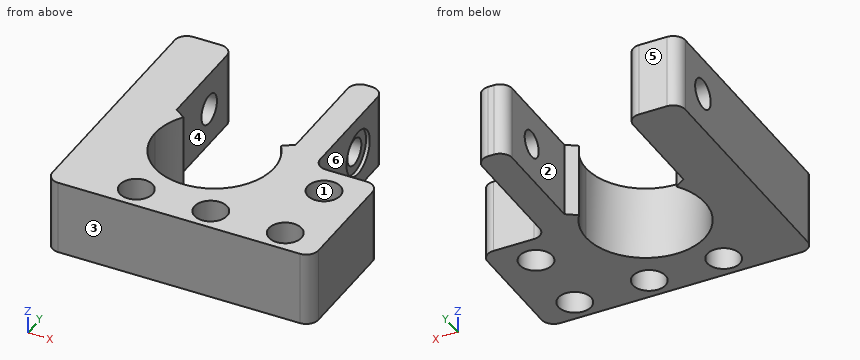
from build123d import *

# Parameters (mm, degrees)
CYLINDER011012_R               = 1.8
CYLINDER011012_DEPTH           = 20
CYLINDER011013_R               = 3
CYLINDER011013_DEPTH           = 20
CYLINDER011010_R               = 2.2
CYLINDER011010_DEPTH           = 100
ARRAY008_X_COUNT               = 3
ARRAY008_X_PITCH               = 10
ARRAY008_Y_COUNT               = 3
ARRAY008_Y_PITCH               = 10
CYLINDER011011_R               = 2
CYLINDER011011_DEPTH           = 20
CYLINDER011014_R               = 8
CYLINDER011014_DEPTH           = 10
CYLINDER011015_W               = 11
CYLINDER011015_H               = 10
CYLINDER011015_ANGLE           = 250
CYLINDER011015_PLACEMENT_ANGLE = 145
PAD_DEPTH                      = 10


with BuildPart() as bolt_hole001:
    # Cylinder011012 → Cylinder011012 (new body)
    with BuildSketch(Plane(origin=(-1, 14, 5), x_dir=(0, 0, -1), z_dir=(1, 0, 0))):
        Circle(CYLINDER011012_R)
    extrude(amount=CYLINDER011012_DEPTH)


with BuildPart() as bolt_head_hole:
    # Cylinder011013 → Cylinder011013 (new body)
    with BuildSketch(Plane(origin=(11.5, 14, 5), x_dir=(0, 0, -1), z_dir=(1, 0, 0))):
        Circle(CYLINDER011013_R)
    extrude(amount=CYLINDER011013_DEPTH)


with BuildPart() as general_insert_hole_array:
    # Cylinder011010 → Cylinder011010 (new body)
    with BuildSketch(Plane.XY):
        Circle(CYLINDER011010_R)
    extrude(amount=CYLINDER011010_DEPTH)

    # Array008 X: general insert hole array ×3


with BuildPart() as general_insert_hole_array_1:
    add(general_insert_hole_array.part)
    with Locations(*[(i * ARRAY008_X_PITCH, 0, 0) for i in range(1, ARRAY008_X_COUNT)]):
        add(general_insert_hole_array.part)

    # Array008 Y: general insert hole array ×3


with BuildPart() as general_insert_hole_array_2:
    add(general_insert_hole_array_1.part)
    with Locations(*[(0, i * ARRAY008_Y_PITCH, 0) for i in range(1, ARRAY008_Y_COUNT)]):
        add(general_insert_hole_array_1.part)


with BuildPart() as general_insert_hole_array_3:
    # Array008 placement: moved
    add(general_insert_hole_array_2.part.moved(Location((-4.5, -21.5, -13))))


with BuildPart() as obj1:
    # Cylinder011011 → Cylinder011011 (new body)
    with BuildSketch(Plane(origin=(-22, 14, 5), x_dir=(0, 0, -1), z_dir=(1, 0, 0))):
        Circle(CYLINDER011011_R)
    extrude(amount=CYLINDER011011_DEPTH)

    # Fusion004: union bolt hole001, bolt head hole, general insert hole array
    add(bolt_hole001.part)
    add(bolt_head_hole.part)
    add(general_insert_hole_array_3.part)


with BuildPart() as cylinder:
    # Cylinder011014 → Cylinder011014 (new body)
    with BuildSketch(Plane.XY):
        Circle(CYLINDER011014_R)
    extrude(amount=CYLINDER011014_DEPTH)


with BuildPart() as cut023015009010:
    # Cylinder011015 → Cylinder011015 (revolve)
    with BuildSketch(Plane.XZ):
        with Locations((5.5, 5)):
            Rectangle(CYLINDER011015_W, CYLINDER011015_H)
    revolve(axis=Axis((0, 0, 0), (0, 0, 1)), revolution_arc=CYLINDER011015_ANGLE)


with BuildPart() as cut023015009010_1:
    # Cylinder011015 placement: moved
    add(cut023015009010.part.rotate(Axis((0, 0, 0), (0, 0, 1)), CYLINDER011015_PLACEMENT_ANGLE))

    # Cut023015009010: cut Cylinder
    add(cylinder.part, mode=Mode.SUBTRACT)


with BuildPart() as shaft_attachment_cut:
    # Sketch002 → Pad (new body)
    with BuildSketch(Plane.XY):
        with BuildLine():
            Line((19.091117, -14.6), (-13.372183, -14.6))
            ThreePointArc((-15, -12.972183), (-14.523223, -14.123223), (-13.372183, -14.6))
            Line((-15, 18.544728), (-15, -12.972183))
            ThreePointArc((-13.372183, 20.172545), (-14.523223, 19.695769), (-15, 18.544728))
            Line((-9.627817, 20.172545), (-13.372183, 20.172545))
            ThreePointArc((-8, 18.544728), (-8.476777, 19.695769), (-9.627817, 20.172545))
            Line((-8, 0), (-8, 18.544728))
            ThreePointArc((-8, 0), (0, -8), (8, 0))
            Line((8, 19.017869), (8, 0))
            ThreePointArc((9.627817, 20.645687), (8.476777, 20.16891), (8, 19.017869))
            Line((10.372183, 20.645687), (9.627817, 20.645687))
            ThreePointArc((12, 19.017869), (11.523223, 20.16891), (10.372183, 20.645687))
            Line((12, 4.227817), (12, 19.017869))
            ThreePointArc((12, 4.227817), (12.476777, 3.076777), (13.627817, 2.6))
            Line((19.091117, 2.6), (13.627817, 2.6))
            ThreePointArc((20.718934, 0.972183), (20.242157, 2.123223), (19.091117, 2.6))
            Line((20.718934, -12.972183), (20.718934, 0.972183))
            ThreePointArc((19.091117, -14.6), (20.242157, -14.123223), (20.718934, -12.972183))
        make_face()
    extrude(amount=PAD_DEPTH)

    # Fusion005: union Cut023015009010
    add(cut023015009010_1.part)

    # Cut023015009009: cut obj1
    add(obj1.part, mode=Mode.SUBTRACT)


solid = shaft_attachment_cut.part
The model under review builds one solid part; all positions refer to its coordinate system, in mm. Face numbers are marked on the shaded views. A direction names the side the tool comes from. Give positions to 0.01 mm unless a question says otherwise; leave off trailing zeros. Order: outer loops, then holes, each group sorted by start corner. A loop starts at its lowest first (then second) coordinate and runs counter-clockwise, first axis right, second up. Notation, with made-up numbers: M 72.25,-40 L 87.25,-40 A7 ccw 87.25,-35 Z; hole C 68.25,32.25 d8. An arc over 180 degrees is marked long. Answer in a Markdown table with one row per item. Add a question column.
1. To check wall thickness, follow line 1 along Y through (x, z) = (15.5, 7); line 2 along X through (y, z) = (14.5, 2); line 3 along X through (y, z) = (16.5, 5). State the ranges of each line that lie inside material, in increasing order.
2. Machinability: for the marked faces 4, 5 and 6, which of the approach directions +Z, -Z, +X, -X, +Y, -Y give a long, thin tool a straight path to every point of the face, cutting with its end or side? Answer none if there is none.
3. Add section B-B on y = 8. State the section outline as (x, z) points.
4. Add section D-D on y = 14. State the section outline as (x, z) points, plus the area to 3 significant figures.
5. Add section A-A on x = 15.5. State the section outline as (y, z) points.
6. For pin 1 Ø3 at (y, z) = (10, 4.5) entering from +X; pin 2 Ø2.5 at (x, z) = (16, 6.5) entering from +Y; pin 3 Ø1.9 at (x, z) = (-11, 7.5) entering from +Y; pin 4 Ø1.8 at (y, z) = (14, 5.5) entering from +X, all flat-tipped, find the tip position at first contact; note any pin that passes through.
7. Mouldability with a two-part tool opening along Y and no side actions: class the marked faces 1, 2 and 3 as released by +Y, released by -Y, zero draft, split by the parting line, or undercut.
The answers:
| question | item | result |
|---|---|---|
| 1 | line 1 | -14.6 to -13.7, -9.3 to -3.7, 0.7 to 2.6 |
| 1 | line 2 | -15 to -8, 8 to 12 |
| 1 | line 3 | -15 to -8, 8 to 11.5 |
| 2 | face 4 | +Z, -Z, +Y |
| 2 | face 5 | +Z, -Z, -X, +Y |
| 2 | face 6 | +Z, -Z, +X, +Y |
| 3 | outline | M -15,0 L -8,0 L -8,10 L -15,10 Z; M 8,0 L 12,0 L 12,10 L 8,10 Z |
| 4 | outline | M -15,0 L -8,0 L -8,3 L -15,3 Z; M -15,7 L -8,7 L -8,10 L -15,10 Z; M 8,0 L 12,0 L 12,2 L 11.5,2 L 11.5,3.2 L 8,3.2 Z; M 8,6.8 L 11.5,6.8 L 11.5,8 L 12,8 L 12,10 L 8,10 Z |
| 4 | area | 66.4 mm2 |
| 5 | outline | M -14.6,0 L -13.7,0 L -13.7,10 L -14.6,10 Z; M -9.3,0 L -3.7,0 L -3.7,10 L -9.3,10 Z; M 0.7,0 L 2.6,0 L 2.6,10 L 0.7,10 Z |
| 6 | pin 1 | x = 12 |
| 6 | pin 2 | y = 2.6 |
| 6 | pin 3 | y = 20.17 |
| 6 | pin 4 | through |
| 7 | face 1 | undercut |
| 7 | face 2 | zero draft |
| 7 | face 3 | released by -Y |
